from build123d import *

# Parameters (mm, degrees)
F0_W     = 101.6
F0_H     = 76.2
F1_DEPTH = 38.1
F2_R     = 6.35
F3_W     = 101.6
F3_H     = 63.5
F4_DEPTH = 9.525
F5_R     = 5.08


with BuildPart() as f1:
    # F0 (on Front) → F1 (new body)
    with BuildSketch(Plane.XZ):
        Rectangle(F0_W, F0_H)
    extrude(amount=F1_DEPTH)

    # F2
    f2_edges = [f1.edges().sort_by_distance(p)[0] for p in [
        (50.8, -19.05, -38.1),
        (50.8, -19.05, 38.1),
        (-50.8, -19.05, 38.1),
        (-50.8, -19.05, -38.1),
    ]]
    fillet(f2_edges, radius=F2_R)

    # F3 (on face) → F4 (join)
    with BuildSketch(Plane.XZ.offset(38.1)):
        Rectangle(F3_W, F3_H)
    extrude(amount=F4_DEPTH)

    # F5
    f5_edges = [f1.edges().sort_by_distance(p)[0] for p in [
        (0, -47.625, 31.75),
        (0, -47.625, -31.75),
    ]]
    fillet(f5_edges, radius=F5_R)


solid = f1.part
For this review, take the finished solid that the model builds, in its own axes (mm). A direction names the side the tool comes from. Give positions to 0.01 mm unless a question says otherwise; leave off trailing zeros. Loops run counter-clockwise (first coordinate to the right, second up) from the corner with the lowest first, then second, coordinate; pieces in that order, holes last. Notation, with made-up numbers: M 60.5,71 L 103.5,71 A34 cw 103.5,108 Z; hole C 61,40.25 d8. An arc over 180 degrees is marked long. Put each result on its own line as item: value. Start each with the question number.
(1) Wall thickness on L1, parallel to Z at x = -41, y = -40.5; L2, parallel to Y at x = 5, z = 32; L3, parallel to X at y = -19.5, z = 32: over which ranges is each line inside the solid? List them lowest first.
(2) Machinability: for faces 1 (the cylindrical face through (-48.99, -19.32, -36.19)), 2 (the flat face through (-1, -40, 31.75)), 3 (the flat face through (-1, -40, -31.75)), which of the approach directions +Z, -Z, +X, -X, +Y, -Y give a long, thin tool a straight path to every point of the face, cutting with its end or side? Answer none if there is none.
(3) Add section A-A, the plane x = 36.5. Write out the cut boundary in (y, z) (3 decimals).
(4) For pin 1 (1.3 mm diameter, centred on x = -10.5, y = -39.5, fed in from +Z); pin 2 (1.3 mm diameter, centred on x = 23.5, y = -41, fed in from -Z); pin 3 (3 mm diameter, centred on x = -19.5, z = -36, fed in from -Y), all flat-tipped, find the tip position at first contact; note any pin that passes through.
Result:
1. L1: z = -31.75 to 31.75
1. L2: y = -38.1 to 0
1. L3: x = -50.8 to 50.8
2. face 1: -Z, -X, +Y, -Y
2. face 2: +Z, +X, -X, -Y
2. face 3: -Z, +X, -X, -Y
3. outline: M -47.625,-26.67 A5.08 ccw -42.545,-31.75 L -38.1,-31.75 L -38.1,-38.1 L 0,-38.1 L 0,38.1 L -38.1,38.1 L -38.1,31.75 L -42.545,31.75 A5.08 ccw -47.625,26.67 Z
4. pin 1: stops at z = 31.75
4. pin 2: stops at z = -31.75
4. pin 3: stops at y = -38.1
